Work out the finished part from the listing and answer in its coordinate system (mm). Round coordinates to 2 decimals unless told otherwise and drop trailing zeros. Loops run counter-clockwise (first coordinate to the right, second up) from the corner with the lowest first, then second, coordinate; pieces in that order, holes last.
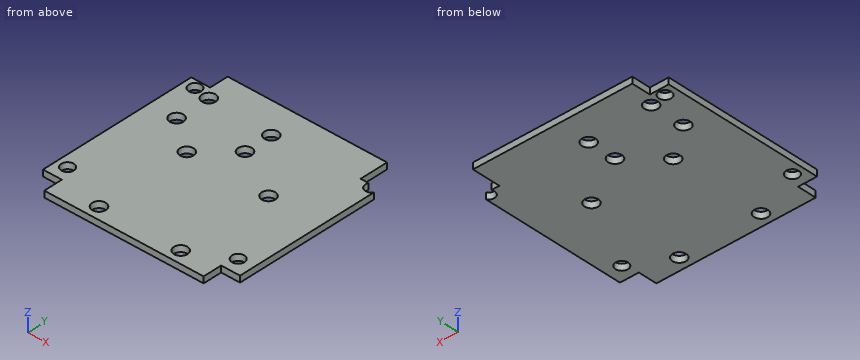
from build123d import *

# Parameters (mm, degrees)
CYLINDER046_R     = 3.25
CYLINDER046_DEPTH = 3
CYLINDER044_R     = 3.25
CYLINDER044_DEPTH = 3
CYLINDER047_R     = 3.25
CYLINDER047_DEPTH = 3
CYLINDER050_R     = 3.25
CYLINDER050_DEPTH = 3
CYLINDER049_R     = 3.25
CYLINDER049_DEPTH = 3
CYLINDER045_R     = 3.25
CYLINDER045_DEPTH = 3
CYLINDER048_R     = 3.25
CYLINDER048_DEPTH = 3
CYLINDER051_R     = 3.25
CYLINDER051_DEPTH = 3
BOX006_W          = 10
BOX006_H          = 10
BOX006_DEPTH      = 3
CYLINDER008_R     = 3
CYLINDER008_DEPTH = 3
CYLINDER009_R     = 3
CYLINDER009_DEPTH = 3
CYLINDER010_R     = 3
CYLINDER010_DEPTH = 3
CYLINDER011_R     = 3
CYLINDER011_DEPTH = 3
BOX003_W          = 12
BOX003_H          = 12
BOX003_DEPTH      = 3
BOX004_W          = 12
BOX004_H          = 12
BOX004_DEPTH      = 3
BOX005_W          = 12
BOX005_H          = 12
BOX005_DEPTH      = 3
BOX002_W          = 12
BOX002_H          = 12
BOX002_DEPTH      = 3
BOX001_W          = 94
BOX001_H          = 94
BOX001_DEPTH      = 3


with BuildPart() as cylinder046:
    # Cylinder046 → Cylinder046 (new body)
    with BuildSketch(Plane(origin=(32.5, 54, 0), x_dir=(1, 0, 0), z_dir=(0, 0, 1))):
        Circle(CYLINDER046_R)
    extrude(amount=CYLINDER046_DEPTH)


with BuildPart() as cylinder044:
    # Cylinder044 → Cylinder044 (new body)
    with BuildSketch(Plane(origin=(32.5, 9, 0), x_dir=(1, 0, 0), z_dir=(0, 0, 1))):
        Circle(CYLINDER044_R)
    extrude(amount=CYLINDER044_DEPTH)


with BuildPart() as cylinder047:
    # Cylinder047 → Cylinder047 (new body)
    with BuildSketch(Plane(origin=(47.25, 68, 0), x_dir=(1, 0, 0), z_dir=(0, 0, 1))):
        Circle(CYLINDER047_R)
    extrude(amount=CYLINDER047_DEPTH)


with BuildPart() as cylinder050:
    # Cylinder050 → Cylinder050 (new body)
    with BuildSketch(Plane(origin=(16, 66.5, 0), x_dir=(1, 0, 0), z_dir=(0, 0, 1))):
        Circle(CYLINDER050_R)
    extrude(amount=CYLINDER050_DEPTH)


with BuildPart() as cylinder049:
    # Cylinder049 → Cylinder049 (new body)
    with BuildSketch(Plane(origin=(47.25, 81.5, 0), x_dir=(1, 0, 0), z_dir=(0, 0, 1))):
        Circle(CYLINDER049_R)
    extrude(amount=CYLINDER049_DEPTH)


with BuildPart() as cylinder045:
    # Cylinder045 → Cylinder045 (new body)
    with BuildSketch(Plane(origin=(71.5, 9, 0), x_dir=(1, 0, 0), z_dir=(0, 0, 1))):
        Circle(CYLINDER045_R)
    extrude(amount=CYLINDER045_DEPTH)


with BuildPart() as cylinder048:
    # Cylinder048 → Cylinder048 (new body)
    with BuildSketch(Plane(origin=(71.5, 54, 0), x_dir=(1, 0, 0), z_dir=(0, 0, 1))):
        Circle(CYLINDER048_R)
    extrude(amount=CYLINDER048_DEPTH)


with BuildPart() as fusion026:
    # Cylinder051 → Cylinder051 (new body)
    with BuildSketch(Plane(origin=(16, 83, 0), x_dir=(1, 0, 0), z_dir=(0, 0, 1))):
        Circle(CYLINDER051_R)
    extrude(amount=CYLINDER051_DEPTH)

    # Fusion026: union Cylinder046, Cylinder044, Cylinder047, Cylinder050, Cylinder049, Cylinder045, Cylinder048
    add(cylinder046.part)
    add(cylinder044.part)
    add(cylinder047.part)
    add(cylinder050.part)
    add(cylinder049.part)
    add(cylinder045.part)
    add(cylinder048.part)


with BuildPart() as cube005:
    # Box006 → Box006 (new body)
    with BuildSketch(Plane(origin=(88, 83.5, 0), x_dir=(1, 0, 0), z_dir=(0, 0, 1))):
        with Locations((5, 5)):
            Rectangle(BOX006_W, BOX006_H)
    extrude(amount=BOX006_DEPTH)


with BuildPart() as main_ata_board_mounting_screws004:
    # Cylinder008 → Cylinder008 (new body)
    with BuildSketch(Plane(origin=(8.3, 18.9, 0), x_dir=(1, 0, 0), z_dir=(0, 0, 1))):
        Circle(CYLINDER008_R)
    extrude(amount=CYLINDER008_DEPTH)


with BuildPart() as main_ata_board_mounting_screws005:
    # Cylinder009 → Cylinder009 (new body)
    with BuildSketch(Plane(origin=(8.3, 84.2, 0), x_dir=(1, 0, 0), z_dir=(0, 0, 1))):
        Circle(CYLINDER009_R)
    extrude(amount=CYLINDER009_DEPTH)


with BuildPart() as main_ata_board_mounting_screws006:
    # Cylinder010 → Cylinder010 (new body)
    with BuildSketch(Plane(origin=(89.6, 19, 0), x_dir=(1, 0, 0), z_dir=(0, 0, 1))):
        Circle(CYLINDER010_R)
    extrude(amount=CYLINDER010_DEPTH)


with BuildPart() as ata_board_mounting_screwholes:
    # Cylinder011 → Cylinder011 (new body)
    with BuildSketch(Plane(origin=(94.5, 82.2, 0), x_dir=(1, 0, 0), z_dir=(0, 0, 1))):
        Circle(CYLINDER011_R)
    extrude(amount=CYLINDER011_DEPTH)

    # Fusion004: union Main ATA Board Mounting Screws004, Main ATA Board Mounting Screws005, Main ATA Board Mounting Screws006
    add(main_ata_board_mounting_screws004.part)
    add(main_ata_board_mounting_screws005.part)
    add(main_ata_board_mounting_screws006.part)


with BuildPart() as cube002:
    # Box003 → Box003 (new body)
    with BuildSketch(Plane(origin=(88, 0, 0), x_dir=(1, 0, 0), z_dir=(0, 0, 1))):
        with Locations((6, 6)):
            Rectangle(BOX003_W, BOX003_H)
    extrude(amount=BOX003_DEPTH)


with BuildPart() as cube003:
    # Box004 → Box004 (new body)
    with BuildSketch(Plane(origin=(88, 88, 0), x_dir=(1, 0, 0), z_dir=(0, 0, 1))):
        with Locations((6, 6)):
            Rectangle(BOX004_W, BOX004_H)
    extrude(amount=BOX004_DEPTH)


with BuildPart() as cube004:
    # Box005 → Box005 (new body)
    with BuildSketch(Plane(origin=(0, 88, 0), x_dir=(1, 0, 0), z_dir=(0, 0, 1))):
        with Locations((6, 6)):
            Rectangle(BOX005_W, BOX005_H)
    extrude(amount=BOX005_DEPTH)


with BuildPart() as fusion003:
    # Box002 → Box002 (new body)
    with BuildSketch(Plane.XY):
        with Locations((6, 6)):
            Rectangle(BOX002_W, BOX002_H)
    extrude(amount=BOX002_DEPTH)

    # Fusion003: union Cube002, Cube003, Cube004
    add(cube002.part)
    add(cube003.part)
    add(cube004.part)


with BuildPart() as backplate_with_nut_recesses:
    # Box001 → Box001 (new body)
    with BuildSketch(Plane(origin=(3, 3, 0), x_dir=(1, 0, 0), z_dir=(0, 0, 1))):
        with Locations((47, 47)):
            Rectangle(BOX001_W, BOX001_H)
    extrude(amount=BOX001_DEPTH)

    # Cut001: cut Fusion003
    add(fusion003.part, mode=Mode.SUBTRACT)

    # Cut002: cut ATA Board mounting screwholes
    add(ata_board_mounting_screwholes.part, mode=Mode.SUBTRACT)

    # Cut003: cut Cube005
    add(cube005.part, mode=Mode.SUBTRACT)

    # Cut014: cut Fusion026
    add(fusion026.part, mode=Mode.SUBTRACT)


solid = backplate_with_nut_recesses.part
Item 1: Section C-C, the plane x = 89.6 is taken. Give the vertices of the cut face in (y, z), plus the area to 4 significant figures.
Item 2: Section D-D, the plane y = 66.5 is taken. Give the vertices of the cut face in (x, z), plus the area to 3 significant figures.
Item 3: Section A-A, the plane z = 2.3 is taken. State how many separate pieces and enclosed holes the cut face has, plus the area to 3 significant figures.
Item 4: Straight lines are drawn through the part: line 1 (Y direction, x = 8.3, z = 2.35); line 2 (Y direction, x = 32.5, z = 1.6); line 3 (X direction, y = 92, z = 0.5). For each, find the intervals that lie inside material, in ascending order.
Item 5: Each of these flat-tipped pins is pushed along its axis until it touches: P1, Ø5, axis at x = 89.6, y = 19, coming from the +Z side; P2, Ø1.5, axis at x = 6, z = 1.5, coming from the +Y side; P3, Ø0.9, axis at x = 8, z = 1.5, coming from the -Y side; P4, Ø1.5, axis at y = 93.5, z = 1.5, coming from the +X side. Where does it stop, or does it pass through?
Item 6: Section B-B, the plane x = 16 is taken. Give the vertices of the cut face in (y, z).
Answer below:
1. outline: (12, 0) - (16, 0) - (16, 3) - (12, 3) - close; (22, 0) - (83.5, 0) - (83.5, 3) - (22, 3) - close
1. area: 196.5 mm2
2. outline: (3, 0) - (12.75, 0) - (12.75, 3) - (3, 3) - close; (19.25, 0) - (44.37, 0) - (44.37, 3) - (19.25, 3) - close; (50.13, 0) - (97, 0) - (97, 3) - (50.13, 3) - close
2. area: 245 mm2
3. separate pieces: 1
3. enclosed holes: 11
3. area: 8,100 mm2
4. line 1: y = 12 to 15.9, 21.9 to 81.2, 87.2 to 88
4. line 2: y = 3 to 5.75, 12.25 to 50.75, 57.25 to 97
4. line 3: x = 12 to 88
5. P1: passes through
5. P2: stops at y = 88
5. P3: stops at y = 12
5. P4: stops at x = 88
6. outline: (3, 0) - (63.25, 0) - (63.25, 3) - (3, 3) - close; (69.75, 0) - (79.75, 0) - (79.75, 3) - (69.75, 3) - close; (86.25, 0) - (97, 0) - (97, 3) - (86.25, 3) - close
